Design review of the part built by this model. Coordinates are the model's own, in mm. A direction names the side the tool comes from. Round coordinates to 2 decimals unless told otherwise and drop trailing zeros. Loops run counter-clockwise (first coordinate to the right, second up) from the corner with the lowest first, then second, coordinate; pieces in that order, holes last. Notation, with made-up numbers: (-15, 1.25) - (26, 1.25) arc R29 ccw to (26, 35.25) - close; hole circle Ø10 at (-0.5, 85.5). An arc over 180 degrees is marked (long way). Use one line per item in the form item = value. Start each with the question number.
(1) For pin 1 (2 mm diameter, centred on x = 43.5, y = -18, fed in from -Z); pin 2 (2.5 mm diameter, centred on y = 1.5, z = 1.5, fed in from -X); pin 3 (0.9 mm diameter, centred on x = -4.5, z = 3.5, fed in from -Y); pin 4 (1.4 mm diameter, centred on x = 30.5, z = 2.5, fed in from -Y), all flat-tipped, find the tip position at first contact; note any pin that passes through.
(2) Wall thickness on probe 1 along Y at (x, z) = (11.5, 3.9); probe 2 along X at (y, z) = (8, 4); probe 3 along X at (y, z) = (15, 1.5): over which ranges is each line inside the solid? List them lowest first. Write a range as [from, to].
(3) The part is to be moulded in two halves that separate along Y. For faces 1 (the flat face through (-7.112, 21, 2)), 2 (the flat face through (19.723, 2.824, 2.254)), 3 (the flat face through (-5, -15.24, 2)), say which applies: released by +Y, released by -Y, zero draft, split by the parting line, or undercut.
(4) We need section B-B, the plane z = 1.15. Give the number of separate pieces and of enclosed holes in the cut face, then the cut area to 3 significant figures.
(5) We need section A-A, the plane x = 8. Write out the cut boundary in (y, z), then the cut area to 3 significant figures.
(6) Machinability: for faces 4 (the flat face through (39.9, -0.2, 2.3)), 5 (the flat face through (-2.032, -11, 2)), 6 (the flat face through (-4, 0, 2)), which of the approach directions +Z, -Z, +X, -X, +Y, -Y give a long, thin tool a straight path to every point of the face, cutting with its end or side? Answer none if there is none.
(7) We need section C-C, the plane x = 43. Write out the cut boundary in (y, z), then the cut area to 3 significant figures.
from build123d import *

# Parameters (mm, degrees)
F0_R     = 2.159
F1_DEPTH = 4.572
F2_R     = 1.01599


# Not quite as in the source:
# - a fillet or chamfer is up to 0.001 mm smaller than in the source, because OpenCascade refuses the exact size


with BuildPart() as f1:
    # F0 (on Top) → F1 (new body)
    with BuildSketch(Plane.XY):
        with BuildLine():
            Line((46.228, 28.956), (-7.112, 28.956))
            Line((-7.112, 28.956), (-7.112, 13.716))
            Line((-7.112, 13.716), (-2.032, 13.716))
            Line((-2.032, 13.716), (-2.032, 21.336))
            Line((-2.032, 21.336), (0, 21.336))
            Line((0, 21.336), (0, 0))
            Line((0, 0), (-7.112, 0))
            Line((-7.112, 0), (-7.112, -15.24))
            Line((-7.112, -15.24), (-2.032, -15.24))
            Line((-2.032, -15.24), (-2.032, -7.62))
            Line((-2.032, -7.62), (0, -7.62))
            Line((0, -7.62), (0, -28.956))
            Line((0, -28.956), (5.08, -28.956))
            Line((5.08, -28.956), (48.5757837838, -14.8692972973))
            ThreePointArc((48.5757837838, -14.8692972973), (52.3905689624, -12.1018683363), (53.848, -7.62))
            Line((53.848, -7.62), (53.848, 21.336))
            ThreePointArc((53.848, 21.336), (51.6161536726, 26.7241536726), (46.228, 28.956))
        make_face()
        Polygon((5.08, -23.6162272727), (5.08, 21.336), (23.9526054243, -17.5040766524), align=None, mode=Mode.SUBTRACT)
        with Locations((46.228, -7.62)):
            Circle(F0_R, mode=Mode.SUBTRACT)
        Polygon((28.8326085769, -15.9236210859), (10.7279551462, 21.336), (42.2585858686, 21.336), align=None, mode=Mode.SUBTRACT)
        with BuildLine():
            Line((46.228, 17.3665858686), (46.228, -2.54))
            ThreePointArc((46.228, -2.54), (41.4862817332, -5.7972252255), (42.8252108486, -11.391926032))
            Line((42.8252108486, -11.391926032), (34.9457461194, -13.9437981318))
            Line((34.9457461194, -13.9437981318), (46.228, 17.3665858686))
        make_face(mode=Mode.SUBTRACT)
        with Locations((46.228, 21.336)):
            Circle(F0_R, mode=Mode.SUBTRACT)
    extrude(amount=F1_DEPTH)

    # F2 (radius 1.016 in the source; OpenCascade refuses exactly that, so slightly less here)
    f2_edges = [f1.edges().sort_by_distance(p)[0] for p in [
        (46.228, 17.366586, 2.286),
        (5.08, 21.336, 2.286),
        (10.727955, 21.336, 2.286),
        (42.258586, 21.336, 2.286),
        (23.952605, -17.504077, 2.286),
        (5.08, -23.616227, 2.286),
        (28.832609, -15.923621, 2.286),
        (46.228, -2.54, 2.286),
        (42.825211, -11.391926, 2.286),
        (34.945746, -13.943798, 2.286),
        (5.08, -28.956, 2.286),
        (0, -28.956, 2.286),
        (0, -7.62, 2.286),
        (-2.032, -7.62, 2.286),
        (-2.032, -15.24, 2.286),
        (-7.112, -15.24, 2.286),
        (0, 21.336, 2.286),
        (-2.032, 13.716, 2.286),
        (-7.112, 13.716, 2.286),
        (-7.112, 0, 2.286),
        (0, 0, 2.286),
        (-2.032, 21.336, 2.286),
        (-7.112, 28.956, 2.286),
    ]]
    fillet(f2_edges, radius=F2_R)


solid = f1.part
Data:
q1.pin_1 = through
q1.pin_2 = -0.35
q1.pin_3 = -15.24
q1.pin_4 = -20.95
q2.probe_1 = [-26.88, -21.54], [8.12, 19.75], [20.87, 28.96]
q2.probe_2 = [0, 5.08], [11.56, 17.21], [37.45, 42.85], [46.23, 53.85]
q2.probe_3 = [-7.11, -2.03], [0, 5.08], [8.16, 13.81], [39.98, 53.85]
q3.face_1 = zero draft
q3.face_2 = undercut
q3.face_3 = released by -Y
q4.separate_pieces = 1
q4.enclosed_holes = 5
q4.area = 1,750 mm^2
q5.outline = (-28.01, 0) - (-22.67, 0) - (-22.67, 4.57) - (-28.01, 4.57) - close; (15.33, 0) - (28.96, 0) - (28.96, 4.57) - (15.33, 4.57) - close
q5.area = 86.7 mm^2
q6.face_4 = +Z, -Z
q6.face_5 = +Z, -Z, -Y
q6.face_6 = +Z, -Z, -X
q7.outline = (-16.68, 0) - (-3.7, 0) - (-3.7, 4.57) - (-16.68, 4.57) - close; (8.41, 0) - (28.96, 0) - (28.96, 4.57) - (8.41, 4.57) - close
q7.area = 153 mm^2
